Source: CAD feature listing. Evaluate the final solid. Frame: model axes, mm. Face numbers are marked on the shaded views. A direction names the side the tool comes from. Give positions to 0.01 mm unless a question says otherwise; leave off trailing zeros. Write each loop counter-clockwise with the first axis right and the second up, starting at its lowest first coordinate (ties: lowest second). Pieces come first, ordered by that corner, then holes. Notation, with made-up numbers: (30.25, 62.5) -> (80.25, 62.5) arc R28 ccw to (80.25, 84.5) -> close; hole circle Ø10 at (-22, 14). An arc over 180 degrees is marked (long way). Use one line per item in the form item = value. Start each with the question number.
(1) Cut plane C-C, the plane x = 0. Output: boundary loops of the cut face in (y, z), and give its area (4 significant figures).
(2) Draft query along Z for the marked faces 3, 4, 5 and 6. Return one class per face: pulls with the +Z half, pulls with the -Z half, needs draft (parallel to the pull), parting line crosses it, or undercut.
(3) Cut plane B-B, the plane z = -52. Output: boundary loops of the cut face in (x, y), and give its area (3 significant figures).
(4) First-contact query: P1, Ø10.5, axis at x = 15, z = 1, coming from the +Y side; P2, Ø8, axis at x = -26, z = -18.5, coming from the +Y side. Flat tips, straight axial feed; report the tip coordinate or a pass-through.
(5) Cut plane A-A, the plane y = 23. Output: boundary loops of the cut face in (x, z).
(6) Material intervals for line 1 along Z through (x, y) = (34, 46); line 2 along X through (y, z) = (35.5, 14); line 3 along Y through (x, z) = (-30, -66.45), sorted ascending. Write a range as from..to.
(7) Set-up query: the marked faces 1 and 2. Return all of +Z, -Z, +X, -X, +Y, -Y with unobstructed straight access to the full face (end or side cutting, diameter ignored); none if empty.
(8) Cut plane D-D, the plane y = 29.5. Output: boundary loops of the cut face in (x, z).
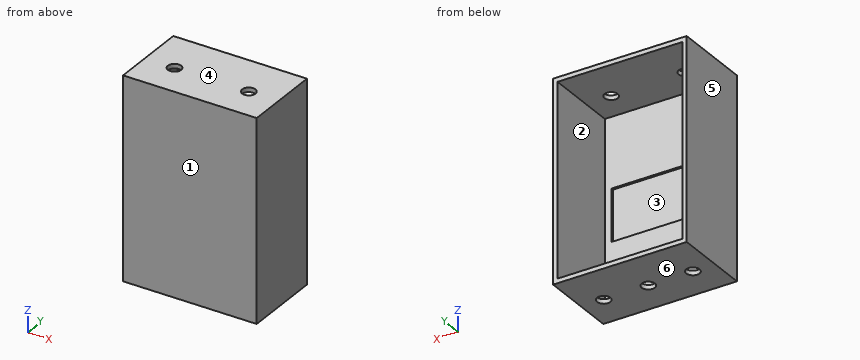
from build123d import *

# Parameters (mm, degrees)
SKETCH1_W           = 90
SKETCH1_H           = 135
BOSS_EXTRUDE1_DEPTH = 3
SKETCH2_W           = 75
SKETCH2_H           = 35
CUT_EXTRUDE1_DEPTH  = 1.5
SKETCH3_W           = 90
SKETCH3_H           = 135
SKETCH3_W_2         = 84
SKETCH3_H_2         = 129
BOSS_EXTRUDE2_DEPTH = 50
SKETCH4_R           = 4.5
CUT_EXTRUDE2_DEPTH  = 3
SKETCH5_R           = 4.5
CUT_EXTRUDE3_DEPTH  = 3


with BuildPart() as part:
    # Sketch1 → Boss-Extrude1 (new body)
    with BuildSketch(Plane(origin=(0, 0, 0), x_dir=(1, 0, 0), z_dir=(0, 1, 0))):
        Rectangle(SKETCH1_W, SKETCH1_H)
    extrude(amount=BOSS_EXTRUDE1_DEPTH)

    # Sketch2 → Cut-Extrude1 (cut)
    with BuildSketch(Plane(origin=(0, 3, 0), x_dir=(1, 0, 0), z_dir=(0, 1, 0))):
        Rectangle(SKETCH2_W, SKETCH2_H)
    extrude(amount=-CUT_EXTRUDE1_DEPTH, mode=Mode.SUBTRACT)

    # Sketch3 → Boss-Extrude2 (add)
    with BuildSketch(Plane(origin=(0, 3, 0), x_dir=(1, 0, 0), z_dir=(0, 1, 0))):
        Rectangle(SKETCH3_W, SKETCH3_H)
        Rectangle(SKETCH3_W_2, SKETCH3_H_2, mode=Mode.SUBTRACT)
    extrude(amount=BOSS_EXTRUDE2_DEPTH)

    # Sketch4 → Cut-Extrude2 (cut)
    with BuildSketch(Plane.XY.offset(67.5)):
        with Locations((-25, 23)):
            Circle(SKETCH4_R)
        with Locations((25, 23)):
            Circle(SKETCH4_R)
    extrude(amount=-CUT_EXTRUDE2_DEPTH, mode=Mode.SUBTRACT)

    # Sketch5 → Cut-Extrude3 (cut)
    with BuildSketch(Plane(origin=(0, 0, -67.5), x_dir=(-1, 0, 0), z_dir=(0, 0, -1))):
        with Locations((-30, 23)):
            Circle(SKETCH5_R)
        with Locations((0, 23)):
            Circle(SKETCH5_R)
        with Locations((30, 23)):
            Circle(SKETCH5_R)
    extrude(amount=-CUT_EXTRUDE3_DEPTH, mode=Mode.SUBTRACT)


solid = part.part
Geometry says:
q1.outline = (0, -67.5) -> (18.5, -67.5) -> (18.5, -64.5) -> (3, -64.5) -> (3, -17.5) -> (1.5, -17.5) -> (1.5, 17.5) -> (3, 17.5) -> (3, 64.5) -> (53, 64.5) -> (53, 67.5) -> (0, 67.5) -> close; (27.5, -67.5) -> (53, -67.5) -> (53, -64.5) -> (27.5, -64.5) -> close
q1.area = 625.5 mm^2
q2.face_3 = undercut
q2.face_4 = pulls with the +Z half
q2.face_5 = needs draft
q2.face_6 = pulls with the -Z half
q3.outline = (-45, 0) -> (45, 0) -> (45, 53) -> (42, 53) -> (42, 3) -> (-42, 3) -> (-42, 53) -> (-45, 53) -> close
q3.area = 570 mm^2
q4.P1 = 1.5
q4.P2 = 3
q5.outline = (-45, -67.5) -> (-34.5, -67.5) -> (-34.5, -64.5) -> (-42, -64.5) -> (-42, 64.5) -> (-29.5, 64.5) -> (-29.5, 67.5) -> (-45, 67.5) -> close; (-25.5, -67.5) -> (-4.5, -67.5) -> (-4.5, -64.5) -> (-25.5, -64.5) -> close; (-20.5, 64.5) -> (20.5, 64.5) -> (20.5, 67.5) -> (-20.5, 67.5) -> close; (4.5, -67.5) -> (25.5, -67.5) -> (25.5, -64.5) -> (4.5, -64.5) -> close; (29.5, 64.5) -> (42, 64.5) -> (42, -64.5) -> (34.5, -64.5) -> (34.5, -67.5) -> (45, -67.5) -> (45, 67.5) -> (29.5, 67.5) -> close
q6.line_1 = -67.5..-64.5, 64.5..67.5
q6.line_2 = -45..-42, 42..45
q6.line_3 = 0..18.5, 27.5..53
q7.face_1 = +Z, -Z, +X, -X, -Y
q7.face_2 = +Y
q8.outline = (-45, -67.5) -> (45, -67.5) -> (45, 67.5) -> (-45, 67.5) -> close; hole (-42, -64.5) -> (42, -64.5) -> (42, 64.5) -> (-42, 64.5) -> close
